from build123d import *

# Parameters (mm, degrees)
BOSS_EXTRUDE1_DEPTH = 0.5
CHAMFER1_SIZE       = 0.5


with BuildPart() as part:
    # Sketch1 → Boss-Extrude1 (new body)
    with BuildSketch(Plane(origin=(0, 0, 0), x_dir=(1, 0, 0), z_dir=(0, 1, 0))):
        Polygon((-78.095165617, -29.786632), (-83.030527551, -38.690260619), (-72.030527551, -38.690260619), (-67.095165617, -29.786632), align=None)
    extrude(amount=BOSS_EXTRUDE1_DEPTH)

    # Chamfer1
    chamfer1_edges = [part.edges().sort_by_distance(p)[0] for p in [
        (-72.595165617, 0.5, 29.786632),
    ]]
    chamfer(chamfer1_edges, length=CHAMFER1_SIZE - 0.0001)  # a hair under: the kernel refuses the full size


solid = part.part
Read the model definition and answer for the solid it produces. Units are mm, in the model's axes. Round coordinates to 2 decimals unless told otherwise and drop trailing zeros. Order: outer loops, then holes, each group sorted by start corner. A loop starts at its lowest first (then second) coordinate and runs counter-clockwise, first axis right, second up. Notation, with made-up numbers: (-33.5, -11.5) - (-29.5, -11.5) arc R29 cw to (-29.5, 21.5) - close; hole circle Ø7 at (-25, 26). An arc over 180 degrees is marked (long way). Use one line per item in the form item = value. Start each with the question number.
(1) Find the intervals of material crossed by line 1 along X through (y, z) = (0.15, 31.75); line 2 along X through (y, z) = (0.2, 32.5); line 3 along Z through (x, y) = (-76, 0.4), in increasing order. Write a range as from..to.
(2) The part is cut by section C-C (z = 32). Give the vertices of the cut face in (x, y).
(3) The part is cut by section B-B (y = 0.3). Give the vertices of the cut face in (x, z), then the cut area to 3 significant figures.
Checked values:
q1.line_1 = -79.18..-68.18
q1.line_2 = -79.6..-68.6
q1.line_3 = 30.19..38.69
q2.outline = (-79.32, 0) - (-68.32, 0) - (-68.32, 0.5) - (-79.32, 0.5) - close
q3.outline = (-83.03, 38.69) - (-78.26, 30.09) - (-67.26, 30.09) - (-72.03, 38.69) - close
q3.area = 94.6 mm^2
